Part model, mm, in its own coordinate system. A direction names the side the tool comes from. Round coordinates to 2 decimals unless told otherwise and drop trailing zeros. Loops run counter-clockwise (first coordinate to the right, second up) from the corner with the lowest first, then second, coordinate; pieces in that order, holes last. Notation, with made-up numbers: M 3.25,87 L 13.25,87 A11 cw 13.25,103 Z; hole C 85.25,19.5 d9. An arc over 180 degrees is marked long. Put each result on its own line as item: value. Start each with the question number.
1) Pull direction X, two halves, no side cores. Call faces 3 (the flat face through (469.9, 121, -100)), 4 (the flat face through (232, 123.825, -74)), 5 (the cylindrical face through (226.56, 122.26, -25.8)), 6 (the flat face through (0, 121, -100)): +X half, -X half, draft (parallel to the pull), parting line (faces both ways), or undercut.
2) Probe line 1 along X through (y, z) = (123.2, -12.7); line 2 along X through (y, z) = (121, -12); line 3 along Y through (x, z) = (304, -67.5) (3 decimals). List the from-to ranges inside material, lowest first.
3) Drop flat-ended pins along their axis: pin 1 Ø6.5 at (x, y) = (460.38, 100.01) entering from +Z (3 decimals); pin 2 Ø5.5 at (x, z) = (460.375, -12.7) entering from -Y. Give the stop position or say it passes through.
4) Slice it at C-C on y = 83. Give the cut face in (x, z) (3 decimals), then the cut area to 3 significant figures.
5) Which spindle directions (+Z, -Z, +X, -X, +Y, -Y) get a long thin tool onto all of the face, cutting with end or side? Do faces 1 (the flat face through (232, 120.65, -72)), 2 (the flat face through (232, 89, -152.4)). Say none if no direction does.
6) Slice it at B-B on z = -121. Give the cut face in (x, y) (3 decimals).
```python
from build123d import *

# Parameters (mm, degrees)
BASE_FLANGE1_DEPTH = 469.9
SKETCH6_R          = 21.9075
CUT_EXTRUDE1_DEPTH = 3.175
SKETCH7_R          = 2.4257
CUT_EXTRUDE2_DEPTH = 510.278313523
SKETCH8_R          = 2.4257
CUT_EXTRUDE3_DEPTH = 510.278313523
SKETCH9_R          = 2.4257
CUT_EXTRUDE4_DEPTH = 510.278313523
FILLET1_R          = 3.175
SKETCH10_W         = 152.4
SKETCH10_H         = 61.9125
CUT_EXTRUDE5_DEPTH = 510.278313523
FILLET2_R          = 3.175


# Sheet-metal steps are written as plain solids
with BuildPart() as part:
    # Sketch1 → Base-Flange1 (new body)
    with BuildSketch(Plane(origin=(0, 0, 0), x_dir=(0, 0, -1), z_dir=(1, 0, 0))):
        with BuildLine():
            Line((0, 0), (146.05, 0))
            ThreePointArc((146.05, 0), (150.540128061, 1.859871939), (152.4, 6.35))
            Line((152.4, 6.35), (152.4, 117.475))
            ThreePointArc((152.4, 117.475), (150.540128061, 121.965128061), (146.05, 123.825))
            Line((146.05, 123.825), (0, 123.825))
            Line((0, 123.825), (0, 120.65))
            Line((0, 120.65), (146.05, 120.65))
            ThreePointArc((146.05, 120.65), (148.29506403, 119.72006403), (149.225, 117.475))
            Line((149.225, 117.475), (149.225, 6.35))
            ThreePointArc((149.225, 6.35), (148.29506403, 4.10493597), (146.05, 3.175))
            Line((146.05, 3.175), (0, 3.175))
            Line((0, 3.175), (0, 0))
        make_face()
    extrude(amount=BASE_FLANGE1_DEPTH)

    # Sketch6 → Cut-Extrude1 (cut)
    with BuildSketch(Plane(origin=(0, 123.825, 0), x_dir=(1, 0, 0), z_dir=(0, 1, 0))):
        with Locations(Location((234.95, 46.0375, 0), (0, 0, 270))):
            Circle(SKETCH6_R)
    extrude(amount=-CUT_EXTRUDE1_DEPTH, mode=Mode.SUBTRACT)

    # Sketch7 → Cut-Extrude2 (cut, through all)
    with BuildSketch(Plane(origin=(0, 123.825, 0), x_dir=(1, 0, 0), z_dir=(0, 1, 0))):
        with Locations(Location((234.95, 12.2555, 0), (0, 0, 270))):
            Circle(SKETCH7_R)
        with Locations(Location((234.95, 79.8195, 0), (0, 0, 270))):
            Circle(SKETCH7_R)
        with Locations(Location((209.55, 12.2555, 0), (0, 0, 270))):
            Circle(SKETCH7_R)
        with Locations(Location((260.35, 12.2555, 0), (0, 0, 270))):
            Circle(SKETCH7_R)
        with Locations(Location((260.35, 79.8195, 0), (0, 0, 270))):
            Circle(SKETCH7_R)
        with Locations(Location((209.55, 79.8195, 0), (0, 0, 270))):
            Circle(SKETCH7_R)
    extrude(amount=-CUT_EXTRUDE2_DEPTH, mode=Mode.SUBTRACT)

    # Sketch8 → Cut-Extrude3 (cut, through all)
    with BuildSketch(Plane(origin=(0, 123.825, 0), x_dir=(1, 0, 0), z_dir=(0, 1, 0))):
        with Locations(Location((460.375, 12.7, 0), (0, 0, 270))):
            Circle(SKETCH8_R)
        with Locations(Location((460.375, 71.4375, 0), (0, 0, 270))):
            Circle(SKETCH8_R)
        with Locations(Location((460.375, 130.175, 0), (0, 0, 270))):
            Circle(SKETCH8_R)
        with Locations(Location((9.525, 130.175, 0), (0, 0, 270))):
            Circle(SKETCH8_R)
        with Locations(Location((9.525, 71.4375, 0), (0, 0, 270))):
            Circle(SKETCH8_R)
        with Locations(Location((9.525, 12.7, 0), (0, 0, 270))):
            Circle(SKETCH8_R)
    extrude(amount=-CUT_EXTRUDE3_DEPTH, mode=Mode.SUBTRACT)

    # Sketch9 → Cut-Extrude4 (cut, through all)
    with BuildSketch(Plane(origin=(0, 0, -152.4), x_dir=(-1, 0, 0), z_dir=(0, 0, -1))):
        with Locations((-460.375, 74.6125)):
            Circle(SKETCH9_R)
        with Locations((-460.375, 49.2125)):
            Circle(SKETCH9_R)
        with Locations((-9.525, 49.2125)):
            Circle(SKETCH9_R)
        with Locations((-9.525, 74.6125)):
            Circle(SKETCH9_R)
        with Locations((-460.375, 100.0125)):
            Circle(SKETCH9_R)
        with Locations((-460.375, 23.8125)):
            Circle(SKETCH9_R)
        with Locations((-9.525, 23.8125)):
            Circle(SKETCH9_R)
        with Locations((-9.525, 100.0125)):
            Circle(SKETCH9_R)
    extrude(amount=-CUT_EXTRUDE4_DEPTH, mode=Mode.SUBTRACT)

    # Fillet1
    fillet1_edges = [part.edges().sort_by_distance(p)[0] for p in [
        (0, 1.5875, 0),
        (0, 122.2375, 0),
        (469.9, 1.5875, 0),
        (469.9, 122.2375, 0),
    ]]
    fillet(fillet1_edges, radius=FILLET1_R)

    # Sketch10 → Cut-Extrude5 (cut, through all)
    with BuildSketch(Plane(origin=(469.9, 0, 0), x_dir=(0, 0, -1), z_dir=(1, 0, 0))):
        with Locations((76.2, 30.95625)):
            Rectangle(SKETCH10_W, SKETCH10_H)
    extrude(amount=-CUT_EXTRUDE5_DEPTH, mode=Mode.SUBTRACT)

    # Fillet2
    fillet2_edges = [part.edges().sort_by_distance(p)[0] for p in [
        (469.9, 61.9125, -150.8125),
        (0, 61.9125, -150.8125),
    ]]
    fillet(fillet2_edges, radius=FILLET2_R)


solid = part.part
```
Recorded:
1. face 3: +X half
1. face 4: draft
1. face 5: undercut
1. face 6: -X half
2. line 1: x = 0 to 7.1, 11.95 to 207.17, 211.93 to 232.57, 237.33 to 257.97, 262.73 to 457.95, 462.8 to 469.9
2. line 2: x = 0 to 7.2, 11.85 to 207.14, 211.96 to 232.54, 237.36 to 257.94, 262.76 to 458.05, 462.7 to 469.9
2. line 3: y = 120.65 to 123.825
3. pin 1: stops at z = -149.225
3. pin 2: stops at y = 120.65
4. outline: M 0,-152.4 L 469.9,-152.4 L 469.9,-149.225 L 0,-149.225 Z
4. area: 1,490 mm2
5. face 1: +Z, +X, -X, -Y
5. face 2: -Z, +X, -X, +Y, -Y
6. outline: M 0,120.65 L 469.9,120.65 L 469.9,123.825 L 0,123.825 Z
